```python
from build123d import *

# Parameters (mm, degrees)
SKETCH1_W           = 36.1
SKETCH1_H           = 36.1
SKETCH1_R           = 1.025
BOSS_EXTRUDE1_DEPTH = 3
SKETCH1_3_W         = 36.1
SKETCH1_3_H         = 36.1
SKETCH1_3_W_2       = 32.1
SKETCH1_3_H_2       = 32.1
BOSS_EXTRUDE2_DEPTH = 8.15
SKETCH2_W           = 17
SKETCH2_H           = 3.65
CUT_EXTRUDE1_DEPTH  = 6
CUT_EXTRUDE2_DEPTH  = 1


with BuildPart() as part:
    # Sketch1 → Boss-Extrude1 (new body)
    with BuildSketch(Plane(origin=(0, 0, 0), x_dir=(1, 0, 0), z_dir=(0, 1, 0))):
        Rectangle(SKETCH1_W, SKETCH1_H)
        with Locations(Location((-14, 14, 0), (0, 0, 270))):
            Circle(SKETCH1_R, mode=Mode.SUBTRACT)
        with Locations(Location((14, 14, 0), (0, 0, 270))):
            Circle(SKETCH1_R, mode=Mode.SUBTRACT)
        with Locations(Location((14, -14, 0), (0, 0, 270))):
            Circle(SKETCH1_R, mode=Mode.SUBTRACT)
        with Locations(Location((-14, -14, 0), (0, 0, 270))):
            Circle(SKETCH1_R, mode=Mode.SUBTRACT)
        with BuildLine():
            Line((-8.64, 2.4), (-8.64, 8.64))
            Line((-8.64, 8.64), (8.64, 8.64))
            Line((8.64, 8.64), (8.64, 2.4))
            Line((8.64, 2.4), (10, 2.4))
            ThreePointArc((10, 2.4), (12.4, 0), (10, -2.4))
            Line((10, -2.4), (8.64, -2.4))
            Line((8.64, -2.4), (8.64, -8.64))
            Line((8.64, -8.64), (-8.64, -8.64))
            Line((-8.64, -8.64), (-8.64, -2.4))
            Line((-8.64, -2.4), (-10, -2.4))
            ThreePointArc((-10, -2.4), (-12.4, 0), (-10, 2.4))
            Line((-10, 2.4), (-8.64, 2.4))
        make_face(mode=Mode.SUBTRACT)
    extrude(amount=BOSS_EXTRUDE1_DEPTH)

    # Sketch1_3 → Boss-Extrude2 (add)
    with BuildSketch(Plane(origin=(0, 0, 0), x_dir=(1, 0, 0), z_dir=(0, 1, 0))):
        Rectangle(SKETCH1_3_W, SKETCH1_3_H)
        Rectangle(SKETCH1_3_W_2, SKETCH1_3_H_2, mode=Mode.SUBTRACT)
    extrude(amount=BOSS_EXTRUDE2_DEPTH)

    # Sketch2 → Cut-Extrude1 (cut)
    with BuildSketch(Plane(origin=(0, 0, -18.05), x_dir=(-1, 0, 0), z_dir=(0, 0, -1))):
        with Locations((0, 6.325)):
            Rectangle(SKETCH2_W, SKETCH2_H)
    extrude(amount=-CUT_EXTRUDE1_DEPTH, mode=Mode.SUBTRACT)

    # Sketch4 → Cut-Extrude2 (cut)
    with BuildSketch(Plane(origin=(0, 8.15, 0), x_dir=(1, 0, 0), z_dir=(0, 1, 0))):
        Polygon((17.05, -17.05), (-17.05, -17.05), (-17.05, 17.05), (-8.5, 17.05), (-8.5, 16.05), (-16.05, 16.05), (-16.05, -16.05), (16.05, -16.05), (16.05, 16.05), (8.5, 16.05), (8.5, 17.05), (17.05, 17.05), align=None)
    extrude(amount=-CUT_EXTRUDE2_DEPTH, mode=Mode.SUBTRACT)


solid = part.part
```
Check sheet for the modelled part. Datum: model origin and axes. Units: mm. A direction names the side the tool comes from. Give positions to 0.01 mm unless a question says otherwise; leave off trailing zeros. Write each loop counter-clockwise with the first axis right and the second up, starting at its lowest first coordinate (ties: lowest second). Pieces come first, ordered by that corner, then holes. Notation, with made-up numbers: (29, 56.5) - (55, 56.5) arc R28 cw to (55, 75.5) - close; hole circle Ø7 at (46.25, 61). An arc over 180 degrees is marked (long way). Answer as a JSON object with one key per item and string values. Group by question number.
1) Access from +Z, -Z, +X, -X, +Y, -Y to the whole of each face (thin tool, end or side, straight path). Record for faces 1 (the face through (0, 4, 18.05)), 2 (the face through (16.05, 5, 0)), 3 (the face through (-8.64, 1, 6)).
2) Sectioned sample at C-C (y = 3.5). Record the cut outline in (x, z).
3) Depth check by flat-ended pin: P1, Ø1.5, axis at x = 11, z = 8, coming from the +Y side. Enter the tip coordinate at first touch or a pass-through.
4) Sectioned sample at B-B (z = 4.5). Record the cut outline in (x, y).
5) Thickness scan on probe 1 along X at (y, z) = (1.3, -14) (3 decimals); probe 2 along Z at (x, y) = (9, 1.25); probe 3 along X at (y, z) = (2.5, 0). Record the ranges inside material, lowest first. Write a range as from..to.
6) Sectioned sample at D-D (x = -14). Record the cut outline in (y, z) (3 decimals).
7) Sectioned sample at A-A (x = 8). Record the cut outline in (y, z).
8) Release check for a two-part mould opening along X. For faces 4 (the face through (0, 3, -18.05)), 5 (the face through (-18.05, 4, 0)), 6 (the face through (18.05, 4, 0)), 7 (the face through (0.1, 7.15, 16.3)) record: pulls with the +X half, pulls with the -X half, needs draft (parallel to the pull), parting line crosses it, or undercut.
Geometry results:
{
 "1": {"face 1": "+Z, +X, -X, +Y, -Y", "face 2": "+Y", "face 3": "+Y, -Y"},
 "2": {"outline": "(-18.05, -18.05) - (18.05, -18.05) - (18.05, 18.05) - (-18.05, 18.05) - close; hole (-16.05, -16.05) - (16.05, -16.05) - (16.05, 16.05) - (-16.05, 16.05) - close"},
 "3": {"P1": "stops at y = 3"},
 "4": {"outline": "(-18.05, 0) - (-8.64, 0) - (-8.64, 3) - (-16.05, 3) - (-16.05, 7.15) - (-17.05, 7.15) - (-17.05, 8.15) - (-18.05, 8.15) - close; (8.64, 0) - (18.05, 0) - (18.05, 8.15) - (17.05, 8.15) - (17.05, 7.15) - (16.05, 7.15) - (16.05, 3) - (8.64, 3) - close"},
 "5": {"probe 1": "x = -18.05..-15.025, -12.975..12.975, 15.025..18.05", "probe 2": "z = -18.05..-2.4, 2.4..18.05", "probe 3": "x = -18.05..-12.4, 12.4..18.05"},
 "6": {"outline": "(0, -18.05) - (8.15, -18.05) - (8.15, -17.05) - (7.15, -17.05) - (7.15, -16.05) - (3, -16.05) - (3, -15.025) - (0, -15.025) - close; (0, -12.975) - (3, -12.975) - (3, 12.975) - (0, 12.975) - close; (0, 15.025) - (3, 15.025) - (3, 16.05) - (7.15, 16.05) - (7.15, 17.05) - (8.15, 17.05) - (8.15, 18.05) - (0, 18.05) - close"},
 "7": {"outline": "(0, -18.05) - (4.5, -18.05) - (4.5, -16.05) - (3, -16.05) - (3, -8.64) - (0, -8.64) - close; (0, 8.64) - (3, 8.64) - (3, 16.05) - (7.15, 16.05) - (7.15, 17.05) - (8.15, 17.05) - (8.15, 18.05) - (0, 18.05) - close"},
 "8": {"face 4": "needs draft", "face 5": "pulls with the -X half", "face 6": "pulls with the +X half", "face 7": "undercut"}
}
